Build history of the part. All positions in model axes, mm. A direction names the side the tool comes from. Round coordinates to 2 decimals unless told otherwise and drop trailing zeros. Order: outer loops, then holes, each group sorted by start corner. A loop starts at its lowest first (then second) coordinate and runs counter-clockwise, first axis right, second up. Notation, with made-up numbers: (86.25, 37.5) -> (118.25, 37.5) arc R13 ccw to (118.25, 59.5) -> close; hole circle Ø7 at (-2, 50). An arc over 180 degrees is marked (long way). Answer as CSV lines item,"result". Start each with the question number.
```python
from build123d import *

# Parameters (mm, degrees)
F1_DEPTH = 5
F2_R     = 0.9
F3_DEPTH = 5.25
F4_R     = 1.7
F5_DEPTH = 3


with BuildPart() as f1:
    # F0 (on Top) → F1 (new body, symmetric)
    with BuildSketch(Plane.XY):
        Polygon((-3, 1.75), (-3, 0), (3, 0), (3, 1.75), (5.5, 1.75), (5.5, 2.25), (2.5, 5.25), (-2.5, 5.25), (-5.5, 2.25), (-5.5, 1.75), align=None)
    extrude(amount=F1_DEPTH, both=True)

    # F2 (on face) → F3 (cut, through all)
    with BuildSketch(Plane.XZ):
        Circle(F2_R)
    extrude(amount=-F3_DEPTH, mode=Mode.SUBTRACT)

    # F4 (on face) → F5 (cut)
    with BuildSketch(Plane(origin=(0, 5.25, 0), x_dir=(-1, 0, 0), z_dir=(0, 1, 0))):
        Circle(F4_R)
    extrude(amount=-F5_DEPTH, mode=Mode.SUBTRACT)


solid = f1.part
```
Q1. Probe L1, parallel to Z at x = 0, y = 1.15; L2, parallel to Z at x = 0, y = 4.05; L3, parallel to X at y = 4.5, z = 1.25. List the from-to ranges inside material, lowest first.
Q2. Slice it at D-D, the plane z = -4. Write the cut outline in (x, y), plus the area to 3 significant figures.
Q3. Slice it at C-C, the plane y = 3.85. Write the cut outline in (x, z).
Q4. Slice it at B-B, the plane x = 0. Write the cut outline in (y, z), plus the area to 4 significant figures.
Q5. Flat gauge pins, fed straight in: pin 1 Ø1 at (y, z) = (0.5, 2) entering from +X; pin 2 Ø3.5 at (x, z) = (1, 0.5) entering from +Y; pin 3 Ø1.9 at (y, z) = (0.5, 2) entering from -X; pin 4 Ø0.8 at (x, z) = (4, -0.5) entering from -Y. Where does each tip first touch, or does it go through?
Q6. Which spindle directions (+Z, -Z, +X, -X, +Y, -Y) get a long thin tool onto all of the face, cutting with end or side? Do faces 1 (the face through (-4, 1.75, 0)), 2 (the face through (3, 1, 0)), 3 (the face through (-1, 2.25, -1)). Say none if no direction does.
Q7. Two-plate mould, pull along Z, no slides. Class faces 4 (the face through (0, 3, 5)), 5 (the face through (-3, 1, 0)), 6 (the face through (0.37, 3.77, -1.66)): +Z half, -Z half, draft (parallel to the pull), parting line (faces both ways), or undercut.
Q8. Slice it at A-A, the plane z = 0. Write the cut outline in (x, y), plus the area to 4 significant figures.
Solutions:
1,L1,"z = -5 to -0.9, 0.9 to 5"
1,L2,"z = -5 to -1.7, 1.7 to 5"
1,L3,"x = -3.25 to -1.15, 1.15 to 3.25"
2,outline,"(-5.5, 1.75) -> (-3, 1.75) -> (-3, 0) -> (3, 0) -> (3, 1.75) -> (5.5, 1.75) -> (5.5, 2.25) -> (2.5, 5.25) -> (-2.5, 5.25) -> (-5.5, 2.25) -> close"
2,area,"40.0 mm2"
3,outline,"(-3.9, -5) -> (3.9, -5) -> (3.9, 5) -> (-3.9, 5) -> close; hole circle Ø3.4 at (0, 0)"
4,outline,"(0, -5) -> (5.25, -5) -> (5.25, -1.7) -> (2.25, -1.7) -> (2.25, -0.9) -> (0, -0.9) -> close; (0, 0.9) -> (2.25, 0.9) -> (2.25, 1.7) -> (5.25, 1.7) -> (5.25, 5) -> (0, 5) -> close"
4,area,"38.25 mm2"
5,pin 1,"stops at x = 3"
5,pin 2,"stops at y = 5.25"
5,pin 3,"stops at x = -3"
5,pin 4,"stops at y = 1.75"
6,face 1,"+Z, -Z, -X, -Y"
6,face 2,"+Z, -Z, +X, -Y"
6,face 3,"+Y"
7,face 4,"+Z half"
7,face 5,"draft"
7,face 6,"undercut"
8,outline,"(-5.5, 1.75) -> (-3, 1.75) -> (-3, 0) -> (-0.9, 0) -> (-0.9, 2.25) -> (-1.7, 2.25) -> (-1.7, 5.25) -> (-2.5, 5.25) -> (-5.5, 2.25) -> close; (0.9, 0) -> (3, 0) -> (3, 1.75) -> (5.5, 1.75) -> (5.5, 2.25) -> (2.5, 5.25) -> (1.7, 5.25) -> (1.7, 2.25) -> (0.9, 2.25) -> close"
8,area,"25.75 mm2"
